```python
from build123d import *

# Parameters (mm, degrees)
BOSS_EXTRU_1_DEPTH         = 3.7
ESQUISSE2_R                = 2
ENL_V_MAT_EXTRU_1_DEPTH    = 47.708671572
R_P_TITION_LIN_AIRE1_COUNT = 6
R_P_TITION_LIN_AIRE1_PITCH = 8
SYM_TRIE1_COPY_1_SKETCH_R  = 2
SYM_TRIE1_COPY_1_DEPTH     = 47.708671572
SYM_TRIE1_COPY_2_SKETCH_R  = 2
SYM_TRIE1_COPY_2_DEPTH     = 47.708671572
SYM_TRIE1_COPY_3_SKETCH_R  = 2
SYM_TRIE1_COPY_3_DEPTH     = 47.708671572
SYM_TRIE1_COPY_4_SKETCH_R  = 2
SYM_TRIE1_COPY_4_DEPTH     = 47.708671572
SYM_TRIE1_COPY_5_SKETCH_R  = 2
SYM_TRIE1_COPY_5_DEPTH     = 47.708671572
ESQUISSE3_W                = 2.3
ESQUISSE3_H                = 15
BOSS_EXTRU_2_DEPTH         = 24
CONG_1_R                   = 2
CONG_1_OF_SYM_TRIE2_R      = 2
ENL_V_MAT_EXTRU_2_DEPTH    = 63.527593909
ESQUISSE5_W                = 0.2
ESQUISSE5_H                = 16.438402163
BOSS_EXTRU_3_DEPTH         = 48


with BuildPart() as part:
    # Esquisse1 → Boss.-Extru.1 (new body)
    with BuildSketch(Plane.XY):
        with BuildLine():
            Line((-20, 39.9), (20, 39.9))
            ThreePointArc((20, 39.9), (22.828427125, 38.728427125), (24, 35.9))
            Line((24, 35.9), (24, -35.9))
            ThreePointArc((24, -35.9), (22.828427125, -38.728427125), (20, -39.9))
            Line((20, -39.9), (-20, -39.9))
            ThreePointArc((-20, -39.9), (-22.828427125, -38.728427125), (-24, -35.9))
            Line((-24, -35.9), (-24, 35.9))
            ThreePointArc((-24, 35.9), (-22.828427125, 38.728427125), (-20, 39.9))
        make_face()
    extrude(amount=BOSS_EXTRU_1_DEPTH)

    # Esquisse2 → Enlèv. mat.-Extru.1 (cut, through all)
    with BuildSketch(Plane.XY.offset(3.7)):
        with Locations((20, 35.97)):
            Circle(ESQUISSE2_R)
        with Locations((20, 27.97)):
            Circle(ESQUISSE2_R)
    enl_v_mat_extru_1 = extrude(amount=-ENL_V_MAT_EXTRU_1_DEPTH, mode=Mode.SUBTRACT)

    # Répétition linéaire1: Enlèv. mat.-Extru.1 ×6
    with Locations(*[(-i * R_P_TITION_LIN_AIRE1_PITCH, 0, 0) for i in range(1, R_P_TITION_LIN_AIRE1_COUNT)]):
        add(enl_v_mat_extru_1, mode=Mode.SUBTRACT)

    # Symétrie1: Enlèv. mat.-Extru.1 across plane
    add(enl_v_mat_extru_1.mirror(Plane.ZX), mode=Mode.SUBTRACT)

    # Symétrie1 copy 1 sketch → Symétrie1 copy 1 (cut, through all)
    with BuildSketch(Plane(origin=(-8, 0, 3.7), x_dir=(1, 0, 0), z_dir=(0, 0, 1))):
        with Locations((20, -35.97)):
            Circle(SYM_TRIE1_COPY_1_SKETCH_R)
        with Locations((20, -27.97)):
            Circle(SYM_TRIE1_COPY_1_SKETCH_R)
    extrude(amount=-SYM_TRIE1_COPY_1_DEPTH, mode=Mode.SUBTRACT)

    # Symétrie1 copy 2 sketch → Symétrie1 copy 2 (cut, through all)
    with BuildSketch(Plane(origin=(-16, 0, 3.7), x_dir=(1, 0, 0), z_dir=(0, 0, 1))):
        with Locations((20, -35.97)):
            Circle(SYM_TRIE1_COPY_2_SKETCH_R)
        with Locations((20, -27.97)):
            Circle(SYM_TRIE1_COPY_2_SKETCH_R)
    extrude(amount=-SYM_TRIE1_COPY_2_DEPTH, mode=Mode.SUBTRACT)

    # Symétrie1 copy 3 sketch → Symétrie1 copy 3 (cut, through all)
    with BuildSketch(Plane(origin=(-24, 0, 3.7), x_dir=(1, 0, 0), z_dir=(0, 0, 1))):
        with Locations((20, -35.97)):
            Circle(SYM_TRIE1_COPY_3_SKETCH_R)
        with Locations((20, -27.97)):
            Circle(SYM_TRIE1_COPY_3_SKETCH_R)
    extrude(amount=-SYM_TRIE1_COPY_3_DEPTH, mode=Mode.SUBTRACT)

    # Symétrie1 copy 4 sketch → Symétrie1 copy 4 (cut, through all)
    with BuildSketch(Plane(origin=(-32, 0, 3.7), x_dir=(1, 0, 0), z_dir=(0, 0, 1))):
        with Locations((20, -35.97)):
            Circle(SYM_TRIE1_COPY_4_SKETCH_R)
        with Locations((20, -27.97)):
            Circle(SYM_TRIE1_COPY_4_SKETCH_R)
    extrude(amount=-SYM_TRIE1_COPY_4_DEPTH, mode=Mode.SUBTRACT)

    # Symétrie1 copy 5 sketch → Symétrie1 copy 5 (cut, through all)
    with BuildSketch(Plane(origin=(-40, 0, 3.7), x_dir=(1, 0, 0), z_dir=(0, 0, 1))):
        with Locations((20, -35.97)):
            Circle(SYM_TRIE1_COPY_5_SKETCH_R)
        with Locations((20, -27.97)):
            Circle(SYM_TRIE1_COPY_5_SKETCH_R)
    extrude(amount=-SYM_TRIE1_COPY_5_DEPTH, mode=Mode.SUBTRACT)

    # Esquisse3 → Boss.-Extru.2 (add, symmetric)
    with BuildSketch(Plane(origin=(0, 0, 0), x_dir=(0, 0, -1), z_dir=(1, 0, 0))):
        with Locations((1.15, 7.5)):
            Rectangle(ESQUISSE3_W, ESQUISSE3_H)
    boss_extru_2 = extrude(amount=BOSS_EXTRU_2_DEPTH, both=True)

    # Congé1
    cong_1_edges = [part.edges().sort_by_distance(p)[0] for p in [
        (0, 15, 0),
    ]]
    fillet(cong_1_edges, radius=CONG_1_R)

    # Symétrie2: Boss.-Extru.2 across plane
    add(boss_extru_2.mirror(Plane.ZX))

    # Congé1 of Symétrie2
    cong_1_of_sym_trie2_edges = [part.edges().sort_by_distance(p)[0] for p in [
        (0, -15, 0),
    ]]
    fillet(cong_1_of_sym_trie2_edges, radius=CONG_1_OF_SYM_TRIE2_R)

    # Esquisse4 → Enlèv. mat.-Extru.2 (cut, through all)
    with BuildSketch(Plane.ZY.offset(24)):
        Polygon((3.7, 18.775233884), (2.2, 17.275233884), (2.2, 14.031809695), (3.7, 12.531809695), align=None)
    enl_v_mat_extru_2 = extrude(amount=-ENL_V_MAT_EXTRU_2_DEPTH, mode=Mode.SUBTRACT)

    # Symétrie3: Enlèv. mat.-Extru.2 across plane
    add(enl_v_mat_extru_2.mirror(Plane.ZX), mode=Mode.SUBTRACT)

    # Esquisse5 → Boss.-Extru.3 (add, through all)
    with BuildSketch(Plane(origin=(24, 0, 0), x_dir=(0, 0, -1), z_dir=(1, 0, 0))):
        with Locations((2.4, -0.002043793)):
            Rectangle(ESQUISSE5_W, ESQUISSE5_H)
    extrude(amount=-BOSS_EXTRU_3_DEPTH)


solid = part.part
```
Read the model definition and answer for the solid it produces. Units are mm, in the model's axes. A direction names the side the tool comes from. Coordinates: 2 decimals unless noted, no trailing zeros. Write each loop counter-clockwise with the first axis right and the second up, starting at its lowest first coordinate (ties: lowest second). Pieces come first, ordered by that corner, then holes. Notation, with made-up numbers: (32.25, 16) -> (82.25, 16) arc R24 ccw to (82.25, 52) -> close; hole circle Ø8 at (-7, 45). An arc over 180 degrees is marked (long way). Answer as a JSON object with one key per item and string values.
Q1. Consider line 1 (Y direction, x = -4, z = 2.05); line 2 (Y direction, x = 0, z = 2.25); line 3 (Y direction, x = 19, z = 2). Determine where each line is inside the solid, lowest interval first. Write a range as [from, to].
The answers:
{"line 1": "y = [-39.9, -37.97], [-33.97, -29.97], [-25.97, 25.97], [29.97, 33.97], [37.97, 39.9]", "line 2": "y = [-39.9, -17.33], [-13.98, 13.98], [17.33, 39.9]", "line 3": "y = [-39.9, -37.7], [-34.24, -29.7], [-26.24, 26.24], [29.7, 34.24], [37.7, 39.9]"}
Q2. The part is cut by section A-A on y = -27.97. Give the vertices of the cut face in (x, z).
The answers:
{"outline": "(-24, 0) -> (-22, 0) -> (-22, 3.7) -> (-24, 3.7) -> close; (-18, 0) -> (-14, 0) -> (-14, 3.7) -> (-18, 3.7) -> close; (-10, 0) -> (-6, 0) -> (-6, 3.7) -> (-10, 3.7) -> close; (-2, 0) -> (2, 0) -> (2, 3.7) -> (-2, 3.7) -> close; (6, 0) -> (10, 0) -> (10, 3.7) -> (6, 3.7) -> close; (14, 0) -> (18, 0) -> (18, 3.7) -> (14, 3.7) -> close; (22, 0) -> (24, 0) -> (24, 3.7) -> (22, 3.7) -> close"}
Q3. The part is cut by section D-D on y = 9. Give the vertices of the cut face in (x, z).
The answers:
{"outline": "(-24, -2.3) -> (24, -2.3) -> (24, 3.7) -> (-24, 3.7) -> close"}
Q4. The part is cut by section B-B on x = -8.5. Give the vertices of the cut face in (y, z).
The answers:
{"outline": "(-39.9, 0) -> (-17, 0) arc R2 cw to (-15, -2) -> (-15, -2.3) -> (-8.22, -2.3) -> (-8.22, -2.5) -> (8.22, -2.5) -> (8.22, -2.3) -> (15, -2.3) -> (15, -2) arc R2 cw to (17, 0) -> (39.9, 0) -> (39.9, 3.7) -> (18.78, 3.7) -> (17.28, 2.2) -> (14.03, 2.2) -> (12.53, 3.7) -> (-12.53, 3.7) -> (-14.03, 2.2) -> (-17.28, 2.2) -> (-18.78, 3.7) -> (-39.9, 3.7) -> close"}
Q5. Determine the mould class of faces 1 (the cylindrical face through (-0.34, -15.6, -0.57)), 2 (the cylindrical face through (-12.434, 26.018, 1.876)), 3 (the flat face through (0, 29, 0)) for opening direction Y: pulls with the +Y half, pulls with the -Y half, needs draft (parallel to the pull), parting line crosses it, or undercut.
The answers:
{"face 1": "pulls with the -Y half", "face 2": "undercut", "face 3": "needs draft"}
Q6. The part is cut by section C-C on z = -0.75. Give the vertices of the cut face in (x, y).
The answers:
{"outline": "(-24, -15.44) -> (24, -15.44) -> (24, 15.44) -> (-24, 15.44) -> close"}
Q7. Flat-ended cylindrical pins translate along their axes: pin 1 Ø3 at (x, y) = (12, -27) entering from -Z; pin 2 Ø1 at (x, z) = (3, -1.5) entering from +Y; pin 3 Ø3.5 at (x, y) = (-4, -27.97) entering from -Z; pin 4 Ø2 at (x, y) = (-8.5, -11) entering from -Z. Find the tip coordinate at first contact, or state that the pin passes through.
The answers:
{"pin 1": "stops at z = 0", "pin 2": "stops at y = 15.27", "pin 3": "passes through", "pin 4": "stops at z = -2.3"}
Q8. A tool of negligible diameter and unlimited length cuts with its end or side. For faces 4 (the cylindrical face through (-20.434, 26.018, 1.876)), 5 (the flat face through (-0.34, -13.29, 2.94)), from which of +Z, -Z, +X, -X, +Y, -Y can it reach the whole face along a straight path? Write none if from no direction.
The answers:
{"face 4": "+Z, -Z", "face 5": "+Z, +X, -X"}
